Input: dimensioned drawing with shaded views. Units: mm. Origin: part minimum x, y, z. Give positions to 0.01 mm unless a question says otherwise; leave off trailing zeros. Loops run counter-clockwise (first coordinate to the right, second up) from the corner with the lowest first, then second, coordinate; pieces in that order, holes last. Notation, with made-up numbers: (41, -28.5) -> (91, -28.5) arc R28 cw to (91, -4.5) -> close; hole circle Ø8 at (23, -25). An arc over 180 degrees is marked (long way). Answer in a Markdown table with one row per item. Add a question column.
1) Section query D-D (x = 82). Return the cut outline in (y, z).
2) Line query: line 1 (X direction, y = 2.05, z = 114); line 2 (X direction, y = 1.25, z = 74.5) (1 decimal); line 3 (Z direction, x = 93, y = 2.95) (1 decimal). Output: solid intervals per line, ascending. Write a range as from..to.
3) Section query B-B (z = 5.2). Return the cut outline in (x, y).
4) First-contact query: P1, Ø0.9, axis at y = 2, z = 2.5, coming from the -X side; P2, Ø1.5, axis at x = 56.5, y = 0.5, coming from the +Z side; P3, Ø4, axis at x = 50, z = 5.2, coming from the -Y side; P4, Ø0.9, axis at y = 1.5, z = 114, coming from the +X side. Flat tips, straight axial feed; report the tip coordinate or a pass-through.
5) Section query A-A (y = 1.5). Return the cut outline in (x, z).
6) Section query C-C (x = 50). Return the cut outline in (y, z).
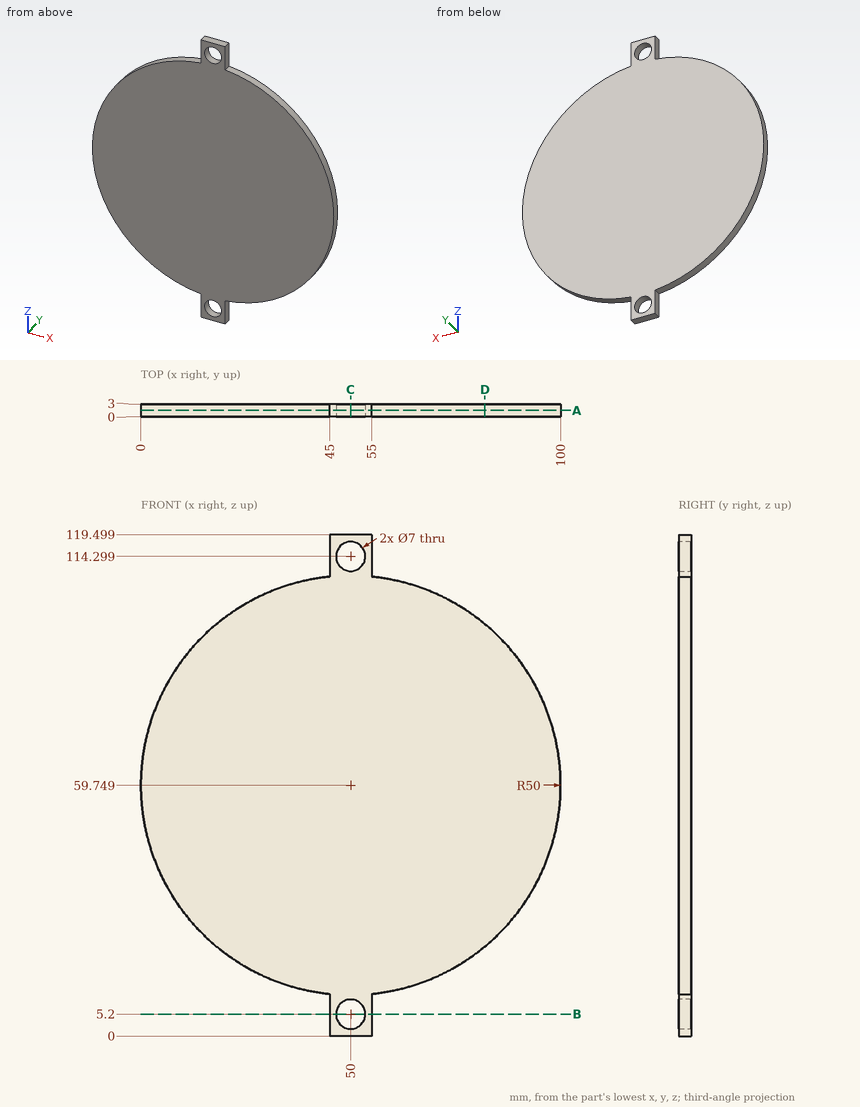
Evaluation:
| question | item | result |
|---|---|---|
| 1 | outline | (0, 21.33) -> (3, 21.33) -> (3, 98.17) -> (0, 98.17) -> close |
| 2 | line 1 | 45..46.51, 53.49..55 |
| 2 | line 2 | 2.2..97.8 |
| 2 | line 3 | 34.2..85.3 |
| 3 | outline | (45, 0) -> (46.5, 0) -> (46.5, 3) -> (45, 3) -> close; (53.5, 0) -> (55, 0) -> (55, 3) -> (53.5, 3) -> close |
| 4 | P1 | x = 45 |
| 4 | P2 | z = 109.42 |
| 4 | P3 | through |
| 4 | P4 | x = 55 |
| 5 | outline | (45, 0) -> (55, 0) -> (55, 10) arc R50 ccw to (55, 109.5) -> (55, 119.5) -> (45, 119.5) -> (45, 109.5) arc R50 ccw to (45, 10) -> close; hole circle Ø7 at (50, 5.2); hole circle Ø7 at (50, 114.3) |
| 6 | outline | (0, 0) -> (3, 0) -> (3, 1.7) -> (0, 1.7) -> close; (0, 8.7) -> (3, 8.7) -> (3, 110.8) -> (0, 110.8) -> close; (0, 117.8) -> (3, 117.8) -> (3, 119.5) -> (0, 119.5) -> close |
